```python
from build123d import *

# Parameters (mm, degrees)
BOSS_EXTRU_1_DEPTH      = 6
ESQUISSE2_W             = 150
ESQUISSE2_H             = 120
BOSS_EXTRU_2_DEPTH      = 6
ESQUISSE3_W             = 6
ESQUISSE3_H             = 50
ESQUISSE3_W_2           = 50
ESQUISSE3_H_2           = 6
ENL_V_MAT_EXTRU_1_DEPTH = 10
ESQUISSE4_W             = 50
ESQUISSE4_H             = 6
ENL_V_MAT_EXTRU_2_DEPTH = 10
ESQUISSE7_W             = 293.706966018
ESQUISSE7_H             = 576.29660199
ENL_V_MAT_EXTRU_4_DEPTH = 10
ESQUISSE8_W             = 6
ESQUISSE8_H             = 40
ESQUISSE8_H_2           = 50
ESQUISSE8_H_3           = 75
BOSS_EXTRU_4_DEPTH      = 6


with BuildPart() as part:
    # Esquisse1 → Boss.-Extru.1 (new body)
    with BuildSketch(Plane.XY):
        Polygon((-50, 335.901139535), (50, 335.901139535), (255.775862069, 10.507079064), (205, -75.642859016), (-205, -75.642859016), (-255.775862069, 10.507079064), align=None)
        with BuildLine():
            Line((-189.319805153, 31.819805153), (-191.794678888, 34.294678888))
            ThreePointArc((-191.794678888, 34.294678888), (-206, 0), (-191.794678888, -34.294678888))
            Line((-191.794678888, -34.294678888), (-189.319805153, -31.819805153))
            ThreePointArc((-189.319805153, -31.819805153), (-202.5, 0), (-189.319805153, 31.819805153))
        make_face(mode=Mode.SUBTRACT)
        with BuildLine():
            Line((-125.680194847, 31.819805153), (-123.205321112, 34.294678888))
            ThreePointArc((-123.205321112, 34.294678888), (-109, 0), (-123.205321112, -34.294678888))
            Line((-123.205321112, -34.294678888), (-125.680194847, -31.819805153))
            ThreePointArc((-125.680194847, -31.819805153), (-112.5, 0), (-125.680194847, 31.819805153))
        make_face(mode=Mode.SUBTRACT)
        with BuildLine():
            Line((-84.319805153, -31.819805153), (-86.794678888, -34.294678888))
            ThreePointArc((-86.794678888, -34.294678888), (-101, 0), (-86.794678888, 34.294678888))
            Line((-86.794678888, 34.294678888), (-84.319805153, 31.819805153))
            ThreePointArc((-84.319805153, 31.819805153), (-97.5, 0), (-84.319805153, -31.819805153))
        make_face(mode=Mode.SUBTRACT)
        with BuildLine():
            Line((-20.680194847, 31.819805153), (-18.205321112, 34.294678888))
            ThreePointArc((-18.205321112, 34.294678888), (-4, 0), (-18.205321112, -34.294678888))
            Line((-18.205321112, -34.294678888), (-20.680194847, -31.819805153))
            ThreePointArc((-20.680194847, -31.819805153), (-7.5, 0), (-20.680194847, 31.819805153))
        make_face(mode=Mode.SUBTRACT)
        with BuildLine():
            Line((20.680194847, -31.819805153), (18.205321112, -34.294678888))
            ThreePointArc((18.205321112, -34.294678888), (4, 0), (18.205321112, 34.294678888))
            Line((18.205321112, 34.294678888), (20.680194847, 31.819805153))
            ThreePointArc((20.680194847, 31.819805153), (7.5, 0), (20.680194847, -31.819805153))
        make_face(mode=Mode.SUBTRACT)
        with BuildLine():
            Line((84.319805153, 31.819805153), (86.794678888, 34.294678888))
            ThreePointArc((86.794678888, 34.294678888), (101, 0), (86.794678888, -34.294678888))
            Line((86.794678888, -34.294678888), (84.319805153, -31.819805153))
            ThreePointArc((84.319805153, -31.819805153), (97.5, 0), (84.319805153, 31.819805153))
        make_face(mode=Mode.SUBTRACT)
        with BuildLine():
            Line((125.680194847, -31.819805153), (123.205321112, -34.294678888))
            ThreePointArc((123.205321112, -34.294678888), (109, 0), (123.205321112, 34.294678888))
            Line((123.205321112, 34.294678888), (125.680194847, 31.819805153))
            ThreePointArc((125.680194847, 31.819805153), (112.5, 0), (125.680194847, -31.819805153))
        make_face(mode=Mode.SUBTRACT)
        with BuildLine():
            Line((189.319805153, 31.819805153), (191.794678888, 34.294678888))
            ThreePointArc((191.794678888, 34.294678888), (206, 0), (191.794678888, -34.294678888))
            Line((191.794678888, -34.294678888), (189.319805153, -31.819805153))
            ThreePointArc((189.319805153, -31.819805153), (202.5, 0), (189.319805153, 31.819805153))
        make_face(mode=Mode.SUBTRACT)
        with BuildLine():
            Line((-139.294678888, 56.63798851), (-136.819805153, 59.112862244))
            ThreePointArc((-136.819805153, 59.112862244), (-150, 90.932667397), (-136.819805153, 122.752472551))
            Line((-136.819805153, 122.752472551), (-139.294678888, 125.227346285))
            ThreePointArc((-139.294678888, 125.227346285), (-153.5, 90.932667397), (-139.294678888, 56.63798851))
        make_face(mode=Mode.SUBTRACT)
        with BuildLine():
            Line((-70.705321112, 56.63798851), (-73.180194847, 59.112862244))
            ThreePointArc((-73.180194847, 59.112862244), (-60, 90.932667397), (-73.180194847, 122.752472551))
            Line((-73.180194847, 122.752472551), (-70.705321112, 125.227346285))
            ThreePointArc((-70.705321112, 125.227346285), (-56.5, 90.932667397), (-70.705321112, 56.63798851))
        make_face(mode=Mode.SUBTRACT)
        with BuildLine():
            Line((-31.819805153, 122.752472551), (-34.294678888, 125.227346285))
            ThreePointArc((-34.294678888, 125.227346285), (-48.5, 90.932667397), (-34.294678888, 56.63798851))
            Line((-34.294678888, 56.63798851), (-31.819805153, 59.112862244))
            ThreePointArc((-31.819805153, 59.112862244), (-45, 90.932667397), (-31.819805153, 122.752472551))
        make_face(mode=Mode.SUBTRACT)
        with BuildLine():
            Line((34.294678888, 56.63798851), (31.819805153, 59.112862244))
            ThreePointArc((31.819805153, 59.112862244), (45, 90.932667397), (31.819805153, 122.752472551))
            Line((31.819805153, 122.752472551), (34.294678888, 125.227346285))
            ThreePointArc((34.294678888, 125.227346285), (48.5, 90.932667397), (34.294678888, 56.63798851))
        make_face(mode=Mode.SUBTRACT)
        with BuildLine():
            Line((73.180194847, 122.752472551), (70.705321112, 125.227346285))
            ThreePointArc((70.705321112, 125.227346285), (56.5, 90.932667397), (70.705321112, 56.63798851))
            Line((70.705321112, 56.63798851), (73.180194847, 59.112862244))
            ThreePointArc((73.180194847, 59.112862244), (60, 90.932667397), (73.180194847, 122.752472551))
        make_face(mode=Mode.SUBTRACT)
        with BuildLine():
            Line((139.294678888, 56.63798851), (136.819805153, 59.112862244))
            ThreePointArc((136.819805153, 59.112862244), (150, 90.932667397), (136.819805153, 122.752472551))
            Line((136.819805153, 122.752472551), (139.294678888, 125.227346285))
            ThreePointArc((139.294678888, 125.227346285), (153.5, 90.932667397), (139.294678888, 56.63798851))
        make_face(mode=Mode.SUBTRACT)
        with BuildLine():
            Line((-84.319805153, 213.685139948), (-86.794678888, 216.160013682))
            ThreePointArc((-86.794678888, 216.160013682), (-101, 181.865334795), (-86.794678888, 147.570655907))
            Line((-86.794678888, 147.570655907), (-84.319805153, 150.045529641))
            ThreePointArc((-84.319805153, 150.045529641), (-97.5, 181.865334795), (-84.319805153, 213.685139948))
        make_face(mode=Mode.SUBTRACT)
        with BuildLine():
            Line((-20.680194847, 213.685139948), (-18.205321112, 216.160013682))
            ThreePointArc((-18.205321112, 216.160013682), (-4, 181.865334795), (-18.205321112, 147.570655907))
            Line((-18.205321112, 147.570655907), (-20.680194847, 150.045529641))
            ThreePointArc((-20.680194847, 150.045529641), (-7.5, 181.865334795), (-20.680194847, 213.685139948))
        make_face(mode=Mode.SUBTRACT)
        with BuildLine():
            Line((20.680194847, 150.045529641), (18.205321112, 147.570655907))
            ThreePointArc((18.205321112, 147.570655907), (4, 181.865334795), (18.205321112, 216.160013682))
            Line((18.205321112, 216.160013682), (20.680194847, 213.685139948))
            ThreePointArc((20.680194847, 213.685139948), (7.5, 181.865334795), (20.680194847, 150.045529641))
        make_face(mode=Mode.SUBTRACT)
        with BuildLine():
            Line((84.319805153, 150.045529641), (86.794678888, 147.570655907))
            ThreePointArc((86.794678888, 147.570655907), (101, 181.865334795), (86.794678888, 216.160013682))
            Line((86.794678888, 216.160013682), (84.319805153, 213.685139948))
            ThreePointArc((84.319805153, 213.685139948), (97.5, 181.865334795), (84.319805153, 150.045529641))
        make_face(mode=Mode.SUBTRACT)
        with BuildLine():
            Line((-31.819805153, 304.617807345), (-34.294678888, 307.09268108))
            ThreePointArc((-34.294678888, 307.09268108), (-48.5, 272.798002192), (-34.294678888, 238.503323305))
            Line((-34.294678888, 238.503323305), (-31.819805153, 240.978197039))
            ThreePointArc((-31.819805153, 240.978197039), (-45, 272.798002192), (-31.819805153, 304.617807345))
        make_face(mode=Mode.SUBTRACT)
        with BuildLine():
            Line((31.819805153, 304.617807345), (34.294678888, 307.09268108))
            ThreePointArc((34.294678888, 307.09268108), (48.5, 272.798002192), (34.294678888, 238.503323305))
            Line((34.294678888, 238.503323305), (31.819805153, 240.978197039))
            ThreePointArc((31.819805153, 240.978197039), (45, 272.798002192), (31.819805153, 304.617807345))
        make_face(mode=Mode.SUBTRACT)
    extrude(amount=BOSS_EXTRU_1_DEPTH)

    # Esquisse2 → Boss.-Extru.2 (add)
    with BuildSketch(Plane.XY.offset(6)):
        with Locations((0, -135.642859016)):
            Rectangle(ESQUISSE2_W, ESQUISSE2_H)
    extrude(amount=-BOSS_EXTRU_2_DEPTH)

    # Esquisse3 → Enlèv. mat.-Extru.1 (cut)
    with BuildSketch(Plane.XY.offset(6)):
        with Locations((-72, -135.642859016)):
            Rectangle(ESQUISSE3_W, ESQUISSE3_H)
        with Locations((0, -192.642859016)):
            Rectangle(ESQUISSE3_W_2, ESQUISSE3_H_2)
        with Locations((72, -135.642859016)):
            Rectangle(ESQUISSE3_W, ESQUISSE3_H)
    extrude(amount=-ENL_V_MAT_EXTRU_1_DEPTH, mode=Mode.SUBTRACT)

    # Esquisse4 → Enlèv. mat.-Extru.2 (cut)
    with BuildSketch(Plane.XY.offset(6)):
        with Locations((-140, -72.642859016)):
            Rectangle(ESQUISSE4_W, ESQUISSE4_H)
        Polygon((-217.693965517, -54.105374496), (-212.524969232, -51.058822772), (-237.912900267, -7.983853732), (-243.081896552, -11.030405456), align=None)
        Polygon((-229.051724138, 52.766047956), (-223.980647871, 49.559151404), (-170.532372009, 134.077089189), (-175.603448276, 137.283985741), align=None)
        Polygon((-71.653061664, 290.43527409), (-76.724137931, 293.642170642), (-130.172413793, 209.124232858), (-125.101337526, 205.917336306), align=None)
        with Locations((0, 332.901139535)):
            Rectangle(ESQUISSE4_W, ESQUISSE4_H)
        with Locations((140, -72.642859016)):
            Rectangle(ESQUISSE4_W, ESQUISSE4_H)
        Polygon((237.912900267, -7.983853732), (243.081896552, -11.030405456), (217.693965517, -54.105374496), (212.524969232, -51.058822772), align=None)
        Polygon((170.532372009, 134.077089189), (175.603448276, 137.283985741), (229.051724138, 52.766047956), (223.980647871, 49.559151404), align=None)
        Polygon((125.101337526, 205.917336306), (130.172413793, 209.124232858), (76.724137931, 293.642170642), (71.653061664, 290.43527409), align=None)
    extrude(amount=-ENL_V_MAT_EXTRU_2_DEPTH, mode=Mode.SUBTRACT)

    # Esquisse7 → Enlèv. mat.-Extru.4 (cut)
    with BuildSketch(Plane.XY.offset(6)):
        with Locations((-146.853483009, 80.947217028)):
            Rectangle(ESQUISSE7_W, ESQUISSE7_H)
    extrude(amount=-ENL_V_MAT_EXTRU_4_DEPTH, mode=Mode.SUBTRACT)

    # Esquisse8 → Boss.-Extru.4 (add)
    with BuildSketch(Plane.XY.offset(6)):
        with Locations((-3, 270.357140984)):
            Rectangle(ESQUISSE8_W, ESQUISSE8_H)
        with Locations((-3, 85.357140984)):
            Rectangle(ESQUISSE8_W, ESQUISSE8_H_2)
        with Locations((-3, -112.142859016)):
            Rectangle(ESQUISSE8_W, ESQUISSE8_H_3)
    extrude(amount=-BOSS_EXTRU_4_DEPTH)


solid = part.part
```
Could you check a few things on this model? Use its own coordinates, in mm. A direction names the side the tool comes from. Coordinates: 2 decimals unless noted, no trailing zeros. Write each loop counter-clockwise with the first axis right and the second up, starting at its lowest first coordinate (ties: lowest second). Pieces come first, ordered by that corner, then holes. Notation, with made-up numbers: M -5,67 L 13,67 A11 ccw 13,73 Z; hole C 85.5,63 d6. An arc over 180 degrees is marked long. Answer as CSV lines item,"result". Start each with the question number.
1) I want a section at D-D, the plane y = 85.5. Please give me the cut outline in (x, z).
2) Please list where these lines run through material, in increasing order: line 1 (Y direction, x = 34.5, z = 5.25); line 2 (Y direction, x = 197, z = 4); line 3 (X direction, y = -28.5, z = 5.25). Write a range as from..to.
3) I want a section at B-B, the plane y = 1. Please give me the cut outline in (x, z).
4) For faces 5 (the cylindrical face through (149.997, 90.438, 2.958)), 6 (the flat face through (211.44, -64.72, 2.96)), which set-ups out of +Z, -Z, +X, -X, +Y, -Y let a thin tool reach every point of the face, with its end or its side?
5) For P1, Ø1.8, axis at x = -2, z = 2, coming from the -Y side; P2, Ø1.8, axis at y = -73, z = 3.5, coming from the -X side; P3, Ø3, axis at y = -175, z = 2.5, coming from the +X side, each with a flat end and sliding along its axis, tell me the tip position at first contact or that it passes through.
6) I want a section at C-C, the plane x = 197.5. Please give me the cut outline in (y, z).
7) I want a section at A-A, the plane x = 40. Please give me the cut outline in (y, z).
8) We'd pull the mould along X, two halves only. Please class faces 1 (the flat face through (242.23, 31.93, 2.96)), 2 (the cylindrical face through (60.003, 90.438, 2.958)), 3 (the flat face through (98, 74, 6)), 4 (the cylindrical face through (109.003, -0.533, 2.958)): +X half, -X half, draft (parallel to the pull), parting line (faces both ways), or undercut.
Data:
1,outline,"M -6,0 L 44.67,0 L 44.67,6 L -6,6 Z; M 48.19,0 L 56.81,0 L 56.81,6 L 48.19,6 Z; M 60.33,0 L 149.67,0 L 149.67,6 L 60.33,6 Z; M 153.19,0 L 201.25,0 L 201.25,6 L 153.19,6 Z"
2,line 1,"y = -195.64..56.84, 62.04..119.82, 125.02..238.71, 243.91..301.69, 306.89..335.9"
2,line 2,"y = -75.64..-28.14, -21.56..21.56, 28.14..92.22"
2,line 3,"x = 0..13.26, 17.68..87.32, 91.74..118.26, 122.68..192.32, 196.74..225.82"
3,outline,"M 0,0 L 4.01,0 L 4.01,6 L 0,6 Z; M 7.51,0 L 97.49,0 L 97.49,6 L 7.51,6 Z; M 100.99,0 L 109.01,0 L 109.01,6 L 100.99,6 Z; M 112.51,0 L 202.49,0 L 202.49,6 L 112.51,6 Z; M 205.99,0 L 250.17,0 L 250.17,6 L 205.99,6 Z"
4,face 5,"+Z, -Z"
4,face 6,"+Z, -Z, +X, -Y"
5,P1,"stops at y = -149.64"
5,P2,"stops at x = 0"
5,P3,"stops at x = 75"
6,outline,"M -75.64,0 L -27.43,0 L -27.43,6 L -75.64,6 Z; M -20.62,0 L 20.62,0 L 20.62,6 L -20.62,6 Z; M 27.43,0 L 91.43,0 L 91.43,6 L 27.43,6 Z"
7,outline,"M -195.64,0 L 63.51,0 L 63.51,6 L -195.64,6 Z; M 70.32,0 L 111.55,0 L 111.55,6 L 70.32,6 Z; M 118.36,0 L 245.37,0 L 245.37,6 L 118.36,6 Z; M 252.18,0 L 293.41,0 L 293.41,6 L 252.18,6 Z; M 300.23,0 L 335.9,0 L 335.9,6 L 300.23,6 Z"
8,face 1,"+X half"
8,face 2,"undercut"
8,face 3,"draft"
8,face 4,"undercut"
